from build123d import *

# Parameters (mm, degrees)
SKETCH1_R           = 1
SKETCH1_W           = 23.5
SKETCH1_H           = 17.5
SKETCH1_W_2         = 6.5
SKETCH1_H_2         = 3.5
BOSS_EXTRUDE1_DEPTH = 1.5


with BuildPart() as part:
    # Sketch1 → Boss-Extrude1 (new, symmetric)
    with BuildSketch(Plane(origin=(0, 0, 0), x_dir=(1, 0, 0), z_dir=(0, 1, 0))):
        with BuildLine():
            Line((33.208457525, 45.046038016), (65.04658306, 48.11170082))
            ThreePointArc((65.04658306, 48.11170082), (67.67262656, 48.730173936), (70.037768086, 50.028141202))
            ThreePointArc((70.037768086, 50.028141202), (81.965379016, 44.719802857), (71.271715852, 37.230348498))
            ThreePointArc((71.271715852, 37.230348498), (68.703419373, 38.05229444), (66.008879463, 38.158108479))
            Line((66.008879463, 38.158108479), (36.823007283, 35.347828626))
            ThreePointArc((36.823007283, 35.347828626), (34.924055904, 34.769058544), (33.4, 33.496956053))
            ThreePointArc((33.4, 33.496956053), (34.472450841, 29.872901682), (35.862619587, 26.358452685))
            ThreePointArc((35.862619587, 26.358452685), (35.793150506, 25.411965218), (34.964285714, 24.949744885))
            ThreePointArc((34.964285714, 24.949744885), (33.219650917, 24.205094625), (32.5, 22.45))
            Line((32.5, 22.45), (32.5, -22.45))
            ThreePointArc((32.5, -22.45), (33.219650917, -24.205094625), (34.964285714, -24.949744885))
            ThreePointArc((34.964285714, -24.949744885), (35.793150506, -25.411965218), (35.862619587, -26.358452685))
            ThreePointArc((35.862619587, -26.358452685), (34.472450841, -29.872901682), (33.4, -33.496956053))
            ThreePointArc((33.4, -33.496956053), (34.924055904, -34.769058544), (36.823007283, -35.347828626))
            Line((36.823007283, -35.347828626), (66.008879463, -38.158108479))
            ThreePointArc((66.008879463, -38.158108479), (68.703419373, -38.05229444), (71.271715852, -37.230348498))
            ThreePointArc((71.271715852, -37.230348498), (81.965379016, -44.719802857), (70.037768086, -50.028141202))
            ThreePointArc((70.037768086, -50.028141202), (67.67262656, -48.730173936), (65.04658306, -48.11170082))
            Line((65.04658306, -48.11170082), (33.208457525, -45.046038016))
            ThreePointArc((33.208457525, -45.046038016), (32.729781285, -45.011516135), (32.25, -45))
            Line((32.25, -45), (-32.25, -45))
            ThreePointArc((-32.25, -45), (-32.729781285, -45.011516135), (-33.208457525, -45.046038016))
            Line((-33.208457525, -45.046038016), (-65.04658306, -48.11170082))
            ThreePointArc((-65.04658306, -48.11170082), (-67.67262656, -48.730173936), (-70.037768086, -50.028141202))
            ThreePointArc((-70.037768086, -50.028141202), (-81.965379016, -44.719802857), (-71.271715852, -37.230348498))
            ThreePointArc((-71.271715852, -37.230348498), (-68.703419373, -38.05229444), (-66.008879463, -38.158108479))
            Line((-66.008879463, -38.158108479), (-36.823007283, -35.347828626))
            ThreePointArc((-36.823007283, -35.347828626), (-34.924055904, -34.769058544), (-33.4, -33.496956053))
            ThreePointArc((-33.4, -33.496956053), (-34.472450841, -29.872901682), (-35.862619587, -26.358452685))
            ThreePointArc((-35.862619587, -26.358452685), (-35.793150506, -25.411965218), (-34.964285714, -24.949744885))
            ThreePointArc((-34.964285714, -24.949744885), (-33.219650917, -24.205094625), (-32.5, -22.45))
            Line((-32.5, -22.45), (-32.5, 22.45))
            ThreePointArc((-32.5, 22.45), (-33.219650917, 24.205094625), (-34.964285714, 24.949744885))
            ThreePointArc((-34.964285714, 24.949744885), (-35.793150506, 25.411965218), (-35.862619587, 26.358452685))
            ThreePointArc((-35.862619587, 26.358452685), (-34.472450841, 29.872901682), (-33.4, 33.496956053))
            ThreePointArc((-33.4, 33.496956053), (-34.924055904, 34.769058544), (-36.823007283, 35.347828626))
            Line((-36.823007283, 35.347828626), (-66.008879463, 38.158108479))
            ThreePointArc((-66.008879463, 38.158108479), (-68.703419373, 38.05229444), (-71.271715852, 37.230348498))
            ThreePointArc((-71.271715852, 37.230348498), (-81.965379016, 44.719802857), (-70.037768086, 50.028141202))
            ThreePointArc((-70.037768086, 50.028141202), (-67.67262656, 48.730173936), (-65.04658306, 48.11170082))
            Line((-65.04658306, 48.11170082), (-33.208457525, 45.046038016))
            ThreePointArc((-33.208457525, 45.046038016), (-32.729781285, 45.011516135), (-32.25, 45))
            Line((-32.25, 45), (32.25, 45))
            ThreePointArc((32.25, 45), (32.729781285, 45.011516135), (33.208457525, 45.046038016))
        make_face()
        with Locations(Location((74.5, 44, 0), (0, 0, 270))):
            Circle(SKETCH1_R, mode=Mode.SUBTRACT)
        with Locations(Location((71.027689375, 46.862351991, 0), (0, 0, 270))):
            Circle(SKETCH1_R, mode=Mode.SUBTRACT)
        with Locations(Location((77.362351991, 47.472310625, 0), (0, 0, 270))):
            Circle(SKETCH1_R, mode=Mode.SUBTRACT)
        with Locations(Location((77.972310625, 41.137648009, 0), (0, 0, 270))):
            Circle(SKETCH1_R, mode=Mode.SUBTRACT)
        with Locations(Location((71.637648009, 40.527689375, 0), (0, 0, 270))):
            Circle(SKETCH1_R, mode=Mode.SUBTRACT)
        with Locations(Location((-71.637648009, 40.527689375, 0), (0, 0, 90))):
            Circle(SKETCH1_R, mode=Mode.SUBTRACT)
        with Locations(Location((-77.972310625, 41.137648009, 0), (0, 0, 90))):
            Circle(SKETCH1_R, mode=Mode.SUBTRACT)
        with Locations(Location((-77.362351991, 47.472310625, 0), (0, 0, 90))):
            Circle(SKETCH1_R, mode=Mode.SUBTRACT)
        with Locations(Location((-71.027689375, 46.862351991, 0), (0, 0, 90))):
            Circle(SKETCH1_R, mode=Mode.SUBTRACT)
        with Locations(Location((-74.5, 44, 0), (0, 0, 90))):
            Circle(SKETCH1_R, mode=Mode.SUBTRACT)
        with Locations(Location((-74.5, -44, 0), (0, 0, 270))):
            Circle(SKETCH1_R, mode=Mode.SUBTRACT)
        with Locations(Location((-71.027689375, -46.862351991, 0), (0, 0, 270))):
            Circle(SKETCH1_R, mode=Mode.SUBTRACT)
        with Locations(Location((-77.362351991, -47.472310625, 0), (0, 0, 270))):
            Circle(SKETCH1_R, mode=Mode.SUBTRACT)
        with Locations(Location((-77.972310625, -41.137648009, 0), (0, 0, 270))):
            Circle(SKETCH1_R, mode=Mode.SUBTRACT)
        with Locations(Location((-71.637648009, -40.527689375, 0), (0, 0, 270))):
            Circle(SKETCH1_R, mode=Mode.SUBTRACT)
        with Locations(Location((71.637648009, -40.527689375, 0), (0, 0, 90))):
            Circle(SKETCH1_R, mode=Mode.SUBTRACT)
        with Locations(Location((77.972310625, -41.137648009, 0), (0, 0, 90))):
            Circle(SKETCH1_R, mode=Mode.SUBTRACT)
        with Locations(Location((77.362351991, -47.472310625, 0), (0, 0, 90))):
            Circle(SKETCH1_R, mode=Mode.SUBTRACT)
        with Locations(Location((71.027689375, -46.862351991, 0), (0, 0, 90))):
            Circle(SKETCH1_R, mode=Mode.SUBTRACT)
        with Locations(Location((74.5, -44, 0), (0, 0, 90))):
            Circle(SKETCH1_R, mode=Mode.SUBTRACT)
        with BuildLine():
            Line((0.54024032, 25.859490032), (18.14024032, 37.158489218))
            ThreePointArc((18.14024032, 37.158489218), (18.559559999, 38.28150419), (17.6, 39))
            Line((17.6, 39), (-17.6, 39))
            ThreePointArc((-17.6, 39), (-18.559559999, 38.28150419), (-18.14024032, 37.158489218))
            Line((-18.14024032, 37.158489218), (-0.54024032, 25.859490032))
            ThreePointArc((-0.54024032, 25.859490032), (0, 25.701000814), (0.54024032, 25.859490032))
        make_face(mode=Mode.SUBTRACT)
        with Locations((14.75, 10.25)):
            Rectangle(SKETCH1_W, SKETCH1_H, mode=Mode.SUBTRACT)
        with Locations((17.75, 23.75)):
            Rectangle(SKETCH1_W_2, SKETCH1_H_2, mode=Mode.SUBTRACT)
        with Locations((-17.75, 23.75)):
            Rectangle(SKETCH1_W_2, SKETCH1_H_2, mode=Mode.SUBTRACT)
        with Locations((-14.75, 10.25)):
            Rectangle(SKETCH1_W, SKETCH1_H, mode=Mode.SUBTRACT)
        with Locations((-14.75, -10.25)):
            Rectangle(SKETCH1_W, SKETCH1_H, mode=Mode.SUBTRACT)
        with Locations((-17.75, -23.75)):
            Rectangle(SKETCH1_W_2, SKETCH1_H_2, mode=Mode.SUBTRACT)
        with BuildLine():
            Line((-18.14024032, -37.158489218), (-0.54024032, -25.859490032))
            ThreePointArc((-0.54024032, -25.859490032), (0, -25.701000814), (0.54024032, -25.859490032))
            Line((0.54024032, -25.859490032), (18.14024032, -37.158489218))
            ThreePointArc((18.14024032, -37.158489218), (18.559559999, -38.28150419), (17.6, -39))
            Line((17.6, -39), (-17.6, -39))
            ThreePointArc((-17.6, -39), (-18.559559999, -38.28150419), (-18.14024032, -37.158489218))
        make_face(mode=Mode.SUBTRACT)
        with Locations((17.75, -23.75)):
            Rectangle(SKETCH1_W_2, SKETCH1_H_2, mode=Mode.SUBTRACT)
        with Locations((14.75, -10.25)):
            Rectangle(SKETCH1_W, SKETCH1_H, mode=Mode.SUBTRACT)
    extrude(amount=BOSS_EXTRUDE1_DEPTH, both=True)


solid = part.part
The listing builds one solid part. Answer for the finished solid, in the listing's coordinates (mm). Coordinates: 2 decimals unless noted, no trailing zeros. Order: outer loops, then holes, each group sorted by start corner. A loop starts at its lowest first (then second) coordinate and runs counter-clockwise, first axis right, second up. Notation, with made-up numbers: (27.25, 82.5) -> (64.25, 82.5) arc R18 ccw to (64.25, 115.5) -> close; hole circle Ø5 at (17.5, 76.25). An arc over 180 degrees is marked (long way). Answer in a Markdown table with one row per item. Add a question column.
Item 1: Find section C-C (y = -0.7). State how many separate pieces and enclosed holes the cut face has, then the cut area to 3 significant figures.
Item 2: Find section B-B (x = -56). Write down the section's boundary in (y, z), then the cut area to 3 significant figures.
Item 3: Find section A-A (z = 30). Write down the section's boundary in (x, y), then the cut area to 3 significant figures.
Item 4: Determine the mould class of faces 1 (the face through (67.708, 0.021, 48.744)), 2 (the face through (51.62, 0.021, -36.773)), 3 (the face through (67.637, 0.021, -48.717)) for opening direction Z: +Z half, -Z half, draft (parallel to the pull), parting line (faces both ways), or undercut.
Item 5: Each of these flat-tipped pins is pushed along its axis until it touches: P1, Ø0.9, axis at y = 0.5, z = 23, coming from the +X side; P2, Ø0.9, axis at x = -15.5, y = 0.5, coming from the -Z side; P3, Ø0.9, axis at y = 0, z = -7.5, coming from the -X side; P4, Ø1.6, axis at x = -71.03, z = -46.86, coming from the +Y side. Where does it stop, or does it pass through?
Item 6: Find the intervals of material crossed by L1, parallel to X at y = 1.2, z = -6.5; L2, parallel to Z at x = -26, y = -0.55; L3, parallel to Z at x = -8, y = 1.3, in increasing order. Write a range as from..to.
Result set:
| question | item | result |
|---|---|---|
| 1 | separate pieces | 1 |
| 1 | enclosed holes | 30 |
| 1 | area | 5,710 mm² |
| 2 | outline | (-1.5, -47.24) -> (1.5, -47.24) -> (1.5, -37.19) -> (-1.5, -37.19) -> close; (-1.5, 37.19) -> (1.5, 37.19) -> (1.5, 47.24) -> (-1.5, 47.24) -> close |
| 2 | area | 60.3 mm² |
| 3 | outline | (-34.43, -1.5) -> (-6.99, -1.5) -> (-6.99, 1.5) -> (-34.43, 1.5) -> close; (6.99, -1.5) -> (34.43, -1.5) -> (34.43, 1.5) -> (6.99, 1.5) -> close |
| 3 | area | 165 mm² |
| 4 | face 1 | +Z half |
| 4 | face 2 | undercut |
| 4 | face 3 | -Z half |
| 5 | P1 | stops at x = 32.71 |
| 5 | P2 | stops at z = -45 |
| 5 | P3 | stops at x = -32.5 |
| 5 | P4 | passes through |
| 6 | L1 | x = -32.5..-26.5, -3..3, 26.5..32.5 |
| 6 | L2 | z = -45..-19, -1.5..1.5, 19..45 |
| 6 | L3 | z = -45..-39, -30.65..-19, -1.5..1.5, 19..30.65, 39..45 |
